Could you check a few things on this model? Use its own coordinates, in mm. Face numbers are marked on the shaded views. A direction names the side the tool comes from. Give positions to 0.01 mm unless a question says otherwise; leave off trailing zeros. Put each result on its own line as item: value.
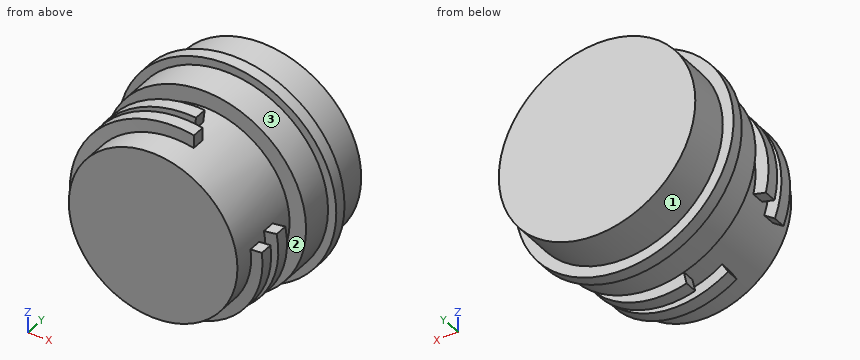
from build123d import *

# Parameters (mm, degrees)
SKETCH1_R           = 20.5
BOSS_EXTRUDE1_DEPTH = 19
SKETCH2_R           = 24.5
BOSS_EXTRUDE2_DEPTH = 8
SKETCH3_R           = 26.5
BOSS_EXTRUDE3_DEPTH = 3
SKETCH4_R           = 23.886443451
BOSS_EXTRUDE4_DEPTH = 10
SWEEP1_PITCH        = 6.35
SWEEP1_HEIGHT       = 1.9685
SWEEP1_RADIUS       = 20.5
SWEEP1_START_ANGLE  = -105
SKETCH10_W          = 6.049698943
SKETCH10_H          = 3.15
SWEEP2_PITCH        = 6.35
SWEEP2_HEIGHT       = 2.2225
SWEEP2_RADIUS       = 20.5
SWEEP2_START_ANGLE  = -111
SKETCH11_W          = 5.521256515
SKETCH11_H          = 3.15
SWEEP3_PITCH        = 6.35
SWEEP3_HEIGHT       = 2.2225
SWEEP3_RADIUS       = 20.5
SWEEP3_START_ANGLE  = 84.999942704
SKETCH18_W          = 6.3
SKETCH18_H          = 3.15
SWEEP4_PITCH        = 6.35
SWEEP4_HEIGHT       = 1.9685
SWEEP4_RADIUS       = 20.5
SWEEP4_START_ANGLE  = 80.999942704
SKETCH19_W          = 6.3
SKETCH19_H          = 3.15


with BuildPart() as part:
    # Sketch1 → Boss-Extrude1 (new body)
    with BuildSketch(Plane(origin=(0, 0, 0), x_dir=(1, 0, 0), z_dir=(0, 1, 0))):
        Circle(SKETCH1_R)
    extrude(amount=BOSS_EXTRUDE1_DEPTH)

    # Sketch2 → Boss-Extrude2 (add)
    with BuildSketch(Plane(origin=(0, 19, 0), x_dir=(1, 0, 0), z_dir=(0, 1, 0))):
        Circle(SKETCH2_R)
    extrude(amount=BOSS_EXTRUDE2_DEPTH)

    # Sketch3 → Boss-Extrude3 (add)
    with BuildSketch(Plane(origin=(0, 27, 0), x_dir=(1, 0, 0), z_dir=(0, 1, 0))):
        Circle(SKETCH3_R)
    extrude(amount=BOSS_EXTRUDE3_DEPTH)

    # Sketch4 → Boss-Extrude4 (add)
    with BuildSketch(Plane(origin=(0, 30, 0), x_dir=(1, 0, 0), z_dir=(0, 1, 0))):
        Circle(SKETCH4_R)
    extrude(amount=BOSS_EXTRUDE4_DEPTH)

    # Sweep1: sweep along a helix
    with BuildLine() as sweep1_path:
        add(Helix(SWEEP1_PITCH, SWEEP1_HEIGHT, SWEEP1_RADIUS, center=(0, 11.25, 0), direction=(0, 1, 0), mode=Mode.PRIVATE).rotate(Axis((0, 11.25, 0), (0, 1, 0)), SWEEP1_START_ANGLE))
    # Sketch10 → Sweep1 (sweep)
    with BuildSketch(Plane.XY):
        with Locations((-20.625150529, 11.420617779)):
            Rectangle(SKETCH10_W, SKETCH10_H)
    sweep(path=sweep1_path.line, is_frenet=True)

    # Sweep2: sweep along a helix
    with BuildLine() as sweep2_path:
        add(Helix(SWEEP2_PITCH, SWEEP2_HEIGHT, SWEEP2_RADIUS, center=(0, 6.25, 0), direction=(0, 1, 0), mode=Mode.PRIVATE).rotate(Axis((0, 6.25, 0), (0, 1, 0)), SWEEP2_START_ANGLE))
    # Sketch11 → Sweep2 (sweep)
    with BuildSketch(Plane.XY.offset(5)):
        with Locations((-20.28419045, 6.826925212)):
            Rectangle(SKETCH11_W, SKETCH11_H)
    sweep(path=sweep2_path.line, is_frenet=True)

    # Sweep3: sweep along a helix
    with BuildLine() as sweep3_path:
        add(Helix(SWEEP3_PITCH, SWEEP3_HEIGHT, SWEEP3_RADIUS, center=(0, 6.25, 0), direction=(0, 1, 0), mode=Mode.PRIVATE).rotate(Axis((0, 6.25, 0), (0, 1, 0)), SWEEP3_START_ANGLE))
    # Sketch18 → Sweep3 (sweep)
    with BuildSketch(Plane.XY):
        with Locations((20.122904995, 6.532252343)):
            Rectangle(SKETCH18_W, SKETCH18_H)
    sweep(path=sweep3_path.line, is_frenet=True)

    # Sweep4: sweep along a helix
    with BuildLine() as sweep4_path:
        add(Helix(SWEEP4_PITCH, SWEEP4_HEIGHT, SWEEP4_RADIUS, center=(0, 11.25, 0), direction=(0, 1, 0), mode=Mode.PRIVATE).rotate(Axis((0, 11.25, 0), (0, 1, 0)), SWEEP4_START_ANGLE))
    # Sketch19 → Sweep4 (sweep)
    with BuildSketch(Plane.XY):
        with Locations((20.5, 11.736280473)):
            Rectangle(SKETCH19_W, SKETCH19_H)
    sweep(path=sweep4_path.line, is_frenet=True)


solid = part.part
1) If I drill on line 1 (Y direction, x = 21, z = -2.5); line 2 (Y direction, x = -20.5, z = 1.5); line 3 (Y direction, x = -15.5, z = 20), over which ranges is the centre line in solid material (lowest first)? Write a range as [from, to].
Filled in:
line 1: y = [5.08, 8.23], [10.28, 13.43], [19, 40]
line 2: y = [5.08, 8.23], [9.92, 13.07], [19, 40]
line 3: y = [27, 30]
2) Which directions (+Z, -Z, +X, -X, +Y, -Y) give clear straight access to the entire face, cutting with the end or side of a thin tool? Please do the marked faces 1, 2 and 3.
Filled in:
face 1: +Y
face 2: none
face 3: -Y
3) I'm going to push flat-ended pins straight in: pin 1 (5 mm diameter, centred on y = 25, z = 6, fed in from +X); pin 2 (1.5 mm diameter, centred on y = 34.5, z = 14.5, fed in from +X); pin 3 (4 mm diameter, centred on y = 14, z = -12.5, fed in from +X). Where does each tip first touch, or does it pass through?
Filled in:
pin 1: stops at x = 26.12
pin 2: stops at x = 19.53
pin 3: stops at x = 21.19
